Work out the finished part from the listing and answer in its coordinate system (mm). A direction names the side the tool comes from. Round coordinates to 2 decimals unless told otherwise and drop trailing zeros. Order: outer loops, then holes, each group sorted by start corner. A loop starts at its lowest first (then second) coordinate and runs counter-clockwise, first axis right, second up. Notation, with made-up numbers: (-17.5, 36) -> (20.5, 36) arc R21 ccw to (20.5, 42) -> close; hole circle Ø9 at (-30.75, 8.5). An arc over 180 degrees is marked (long way). Use a Markdown table: item, result. Add a question column.
Item 1: A tool of negligible diameter and unlimited length cuts with its end or side. For faces 5 (the flat face through (11.04, 2.08, 7.95)), 6 (the flat face through (6, 5.5, 9)), 7 (the flat face through (6, 0, 8)), from which of +Z, -Z, +X, -X, +Y, -Y can it reach the whole face along a straight path? Write none if from no direction.
Item 2: For a pull along X with two mould halves and no side action, classify faces 1 (the flat face through (5.9, 3.6, 1.676)), 2 (the flat face through (6, 1, 15.676)), 3 (the flat face through (11.985, 4, 8)), 4 (the flat face through (0.97, 2.05, 7.95)) as +X half, -X half, draft (parallel to the pull), parting line (faces both ways), or undercut.
Item 3: A cutting plane is placed at B-B, the plane z = 3.25. Give the number of separate pieces and of enclosed holes in the cut face, plus the area to 3 significant figures.
Item 4: Find the intervals of material crossed by L1, parallel to Y at x = 7.25, z = 11.75; L2, parallel to Y at x = 0.75, z = 8; L3, parallel to Y at x = 3, z = 14.75, in increasing order. Write a range as [from, to].
Item 5: A cutting plane is placed at A-A, the plane x = 3.5. Determine the outline of the cut face in (y, z).
Item 6: A cutting plane is placed at C-C, the plane y = 3.5. Determine the outline of the cut face in (x, z), plus the area to 3 significant figures.
Item 7: Flat-ended cylindrical pins translate along their axes: P1, Ø0.6, axis at y = 6, z = 14, coming from the -X side; P2, Ø0.5, axis at x = 9.5, y = 4.5, coming from the +Z side; P3, Ø1.5, axis at x = 10.5, z = 6, coming from the +Y side. Find the tip coordinate at first contact, or state that the pin passes through.
Autodesk Inventor part; units mm, degrees
ref_plane "YZ Plane" through (0, 0, 0) normal (1, 0, 0) x (0, 1, 0)
ref_plane "XZ Plane" through (0, 0, 0) normal (0, 1, 0) x (-1, 0, 0)
ref_plane "XY Plane" through (0, 0, 0) normal (0, 0, 1) x (1, 0, 0)
sketch "Sketch1" plane through (0, 0, 0) normal (0, 1, 0) x (-1, 0, 0)
  line L0 (0, 0) -> (0, 15.676)
  line L1 (0, 15.676) -> (-11.985, 15.676)
  line L2 (-11.985, 15.676) -> (-11.985, 0)
  line L3 (-11.985, 0) -> (0, 0)
  dimension "d1" = 15.676
  dimension "d2" = 11.985
extrude "Extrusion1" add sketch "Sketch1" along normal blind 6
sketch "Sketch2" plane through (0, 0, 15.676) normal (0, 0, 1) x (1, 0, 0)
  line L0 (11.985, 0) -> (0, 0)
  line L1 (0, 0) -> (0, 6)
  line L2 (11.985, 0) -> (11.985, 6)
  line L3 (1.7246, 1) -> (10.26, 1)
  line L4 (1.7246, 1) -> (0.1886, 3.1326)
  line L5 (11.7964, 3.1326) -> (10.26, 1)
  line L6 (0, 3.717) -> (0, 5)
  line L7 (1, 6) -> (10.985, 6)
  line L8 (11.985, 5) -> (11.985, 3.7171)
  line L9 (1.7246, 1) -> (0, 1)
  line L10 (10.26, 1) -> (11.985, 1)
  arc A0 (1, 6) -> (0, 5) centre (1, 5) ccw
  arc A1 (11.985, 5) -> (10.985, 6) centre (10.985, 5) ccw
  line L11 (1, 6) -> (10.985, 6)
  line L12 (11.985, 6) -> (0, 6)
  arc A2 (0, 3.717) -> (0.1886, 3.1326) centre (1, 3.717) ccw
  arc A3 (11.7964, 3.1326) -> (11.985, 3.7171) centre (10.985, 3.7171) ccw
  line L13 (0, 5) -> (0.5, 5)
  arc A4 (1.5, 5.5) -> (0.5, 4.5) centre (1.5, 4.5) ccw
  line L14 (1.5, 5.5) -> (10.485, 5.5)
  arc A5 (11.485, 4.5) -> (10.485, 5.5) centre (10.485, 4.5) ccw
  line L15 (0.5, 4.5) -> (0.5, 3.8784)
  line L16 (0.6886, 3.2939) -> (1.6205, 2)
  arc A6 (0.5, 3.8784) -> (0.6886, 3.2939) centre (1.5, 3.8784) ccw
  line L17 (11.2964, 3.2939) -> (10.3641, 1.9999)
  line L18 (9.5528, 1.5845) -> (2.4319, 1.5845)
  line L19 (11.485, 4.5) -> (11.485, 3.8785)
  arc A7 (11.2964, 3.2939) -> (11.485, 3.8785) centre (10.485, 3.8785) ccw
  arc A8 (1.6205, 2) -> (2.4319, 1.5845) centre (2.4319, 2.5845) ccw
  arc A9 (9.5528, 1.5845) -> (10.3641, 1.9999) centre (9.5528, 2.5845) ccw
  line L20 (1.5, 4.5) -> (10.485, 4.5)
  line L21 (10.485, 4.5) -> (10.485, 3.8785)
  line L22 (10.485, 3.8785) -> (1.5, 3.8785)
  line L23 (1.5, 3.8785) -> (1.5, 4.5)
  line L24 (1.866, 4.5) -> (2.2834, 4.5)
  line L25 (2.2834, 4.5) -> (2.2834, 3.8785)
  line L26 (2.2834, 3.8785) -> (1.866, 3.8785)
  line L27 (1.866, 3.8785) -> (1.866, 4.5)
  line L28 (3.2834, 4.5) -> (3.2834, 3.8785)
  line L29 (2.866, 4.5) -> (3.2834, 4.5)
  line L30 (2.866, 3.8785) -> (2.866, 4.5)
  line L31 (3.2834, 3.8785) -> (2.866, 3.8785)
  line L32 (4.2834, 4.5) -> (4.2834, 3.8785)
  line L33 (3.866, 4.5) -> (4.2834, 4.5)
  line L34 (3.866, 3.8785) -> (3.866, 4.5)
  line L35 (4.2834, 3.8785) -> (3.866, 3.8785)
  line L36 (5.2834, 4.5) -> (5.2834, 3.8785)
  line L37 (4.866, 4.5) -> (5.2834, 4.5)
  line L38 (4.866, 3.8785) -> (4.866, 4.5)
  line L39 (5.2834, 3.8785) -> (4.866, 3.8785)
  line L40 (6.2834, 4.5) -> (6.2834, 3.8785)
  line L41 (5.866, 4.5) -> (6.2834, 4.5)
  line L42 (5.866, 3.8785) -> (5.866, 4.5)
  line L43 (6.2834, 3.8785) -> (5.866, 3.8785)
  line L44 (7.2834, 4.5) -> (7.2834, 3.8785)
  line L45 (6.866, 4.5) -> (7.2834, 4.5)
  line L46 (6.866, 3.8785) -> (6.866, 4.5)
  line L47 (7.2834, 3.8785) -> (6.866, 3.8785)
  line L48 (8.2834, 4.5) -> (8.2834, 3.8785)
  line L49 (7.866, 4.5) -> (8.2834, 4.5)
  line L50 (7.866, 3.8785) -> (7.866, 4.5)
  line L51 (8.2834, 3.8785) -> (7.866, 3.8785)
  line L52 (9.2834, 4.5) -> (9.2834, 3.8785)
  line L53 (8.866, 4.5) -> (9.2834, 4.5)
  line L54 (8.866, 3.8785) -> (8.866, 4.5)
  line L55 (9.2834, 3.8785) -> (8.866, 3.8785)
  line L56 (10.2834, 4.5) -> (10.2834, 3.8785)
  line L57 (9.866, 4.5) -> (10.2834, 4.5)
  line L58 (9.866, 3.8785) -> (9.866, 4.5)
  line L59 (10.2834, 3.8785) -> (9.866, 3.8785)
  line L60 (0, 6) -> (1, 6)
  line L61 (0, 6) -> (0, 5)
  line L62 (10.985, 6) -> (11.985, 6)
  line L63 (11.985, 6) -> (11.985, 5)
  line L64 (11.985, 3.7171) -> (11.985, 1)
  line L65 (0, 3.717) -> (0, 1)
  point P0 (0, 3.3944)
  point P1 (11.985, 3.3944)
  dimension "d7" = 1
  dimension "d8" = 1
  dimension "d9" = 1
  dimension "d12" = 1
  dimension "d14" = 1
  dimension "d16" = 1
  dimension "d18" = 1
  dimension "d19" = 1
  dimension "d20" = 1
  dimension "d23" = 1
extrude "Extrusion2" cut sketch "Sketch2" against normal blind 16 contours L10 L5 A3 L2 | L1 A2 L4 L9 | A1 L12 L2 | L1 L12 A0
extrude "Extrusion3" cut sketch "Sketch2" against normal blind 14 contours L14 A5 L19 A7 L17 A9 L18 A8 L16 A6 L15 A4
extrude "Extrusion4" cut sketch "Sketch2" against normal blind 4 contours L20 L27 L22 L23 | L20 L30 L22 L25 | L20 L34 L22 L28 | L20 L38 L22 L32 | L20 L42 L22 L36 | L20 L46 L22 L40 | L20 L50 L22 L44 | L20 L54 L22 L48 | L20 L58 L22 L52 | L20 L21 L22 L56
extrude "Extrusion5" cut sketch "Sketch2" against normal blind 3 contours L20 L25 L22 L27 | L20 L28 L22 L30 | L20 L34 L22 L28 | L20 L32 L22 L34 | L20 L38 L22 L32 | L20 L36 L22 L38 | L20 L42 L22 L36 | L20 L40 L22 L42 | L20 L46 L22 L40 | L20 L44 L22 L46 | L20 L50 L22 L44 | L20 L48 L22 L50 | L20 L54 L22 L48 | L20 L52 L22 L54 | L20 L58 L22 L52 | L20 L56 L22 L58 | L20 L21 L22 L56
sketch "Sketch3" plane through (0, 6, 0) normal (0, 1, 0) x (1, 0, 0)
  line L0 (2.4319, -10.8223) -> (2.4319, -13.627)
  line L1 (2.4319, -15.676) -> (2.4319, -1.676)
  line L2 (2.4319, -10.8223) -> (2.4319, -13.627)
  line L3 (2.4319, -13.627) -> (3.7319, -13.627)
  line L4 (3.7319, -13.627) -> (3.7319, -10.8223)
  line L5 (3.7319, -10.8223) -> (2.4319, -10.8223)
  line L6 (9.5528, -15.676) -> (9.5528, -1.676)
  line L7 (9.5528, -10.8223) -> (9.5528, -13.627)
  line L8 (9.5528, -13.627) -> (8.2528, -13.627)
  line L9 (8.2528, -13.627) -> (8.2528, -10.8223)
  line L10 (8.2528, -10.8223) -> (9.5528, -10.8223)
  line L11 (2.4319, -13.627) -> (3.7319, -13.627)
  line L12 (3.7319, -13.627) -> (3.7319, -14.3676)
  line L13 (3.7319, -14.3676) -> (2.4319, -14.3676)
  line L14 (2.4319, -14.3676) -> (2.4319, -13.627)
  line L15 (8.2528, -13.627) -> (9.5528, -13.627)
  line L16 (9.5528, -13.627) -> (9.5528, -14.3676)
  line L17 (9.5528, -14.3676) -> (8.2528, -14.3676)
  line L18 (8.2528, -14.3676) -> (8.2528, -13.627)
  point P0 (0, 0)
  dimension "d38" = 1.3
  dimension "d40" = 1.3
extrude "Extrusion6" cut sketch "Sketch3" against normal blind 1 contours L5 L4 L3 L0 | L8 L9 L10 L6
extrude "Extrusion7" add sketch "Sketch3" along normal blind 0.5 contours L3 L12 L13 L1 | L17 L18 L8 L6
chamfer "Chamfer1" distance 0.2 angle 45 3 edges at (1.5, 4.1892, 11.676) (10.485, 4.1892, 11.676) (8.9028, 6.5, 13.627)
chamfer "Chamfer2" distance 0.2 angle 45 1 edges at (3.0819, 6.5, 13.627)
chamfer "Chamfer3" distance 0.2 angle 45 2 edges at (3.0819, 6, 10.8223) (8.9028, 6, 10.8223)
properties part number "Port 3"
Reported:
| question | item | result |
|---|---|---|
| 1 | face 5 | +Z, -Z, +X |
| 1 | face 6 | +Z |
| 1 | face 7 | +Z, -Z, +X, -X, -Y |
| 2 | face 1 | undercut |
| 2 | face 2 | draft |
| 2 | face 3 | +X half |
| 2 | face 4 | -X half |
| 3 | separate pieces | 2 |
| 3 | enclosed holes | 1 |
| 3 | area | 33.2 mm² |
| 4 | L1 | [0, 1.58], [3.88, 4.5], [5.5, 6] |
| 4 | L2 | [0, 1], [2.35, 3.21], [5.16, 5.97] |
| 4 | L3 | [0, 1.58], [5.5, 6] |
| 5 | outline | (0, 0) -> (6, 0) -> (6, 10.62) -> (5.8, 10.82) -> (5.5, 10.82) -> (5.5, 1.68) -> (4.5, 1.68) -> (4.5, 11.68) -> (3.88, 11.68) -> (3.88, 1.68) -> (1.58, 1.68) -> (1.58, 15.68) -> (0, 15.68) -> close; (5.5, 13.63) -> (6.3, 13.63) -> (6.5, 13.83) -> (6.5, 14.37) -> (6, 14.37) -> (6, 15.68) -> (5.5, 15.68) -> close |
| 6 | outline | (0.02, 0) -> (11.96, 0) -> (11.96, 15.68) -> (11.41, 15.68) -> (11.41, 1.68) -> (0.57, 1.68) -> (0.57, 15.68) -> (0.02, 15.68) -> close |
| 6 | area | 35.4 mm² |
| 7 | P1 | x = 0.29 |
| 7 | P2 | z = 12.68 |
| 7 | P3 | y = 6 |
